For this review, use the dimensioned drawing (mm, ordinates from the lowest corner) and the shaded views. A direction names the side the tool comes from. Coordinates: 2 decimals unless noted, no trailing zeros. Order: outer loops, then holes, each group sorted by start corner. A loop starts at its lowest first (then second) coordinate and runs counter-clockwise, first axis right, second up. Notation, with made-up numbers: M 18.25,15.25 L 53.25,15.25 A21 ccw 53.25,36.25 Z; hole C 62.25,12 d2. An arc over 180 degrees is marked long. One line per item, written item: value.
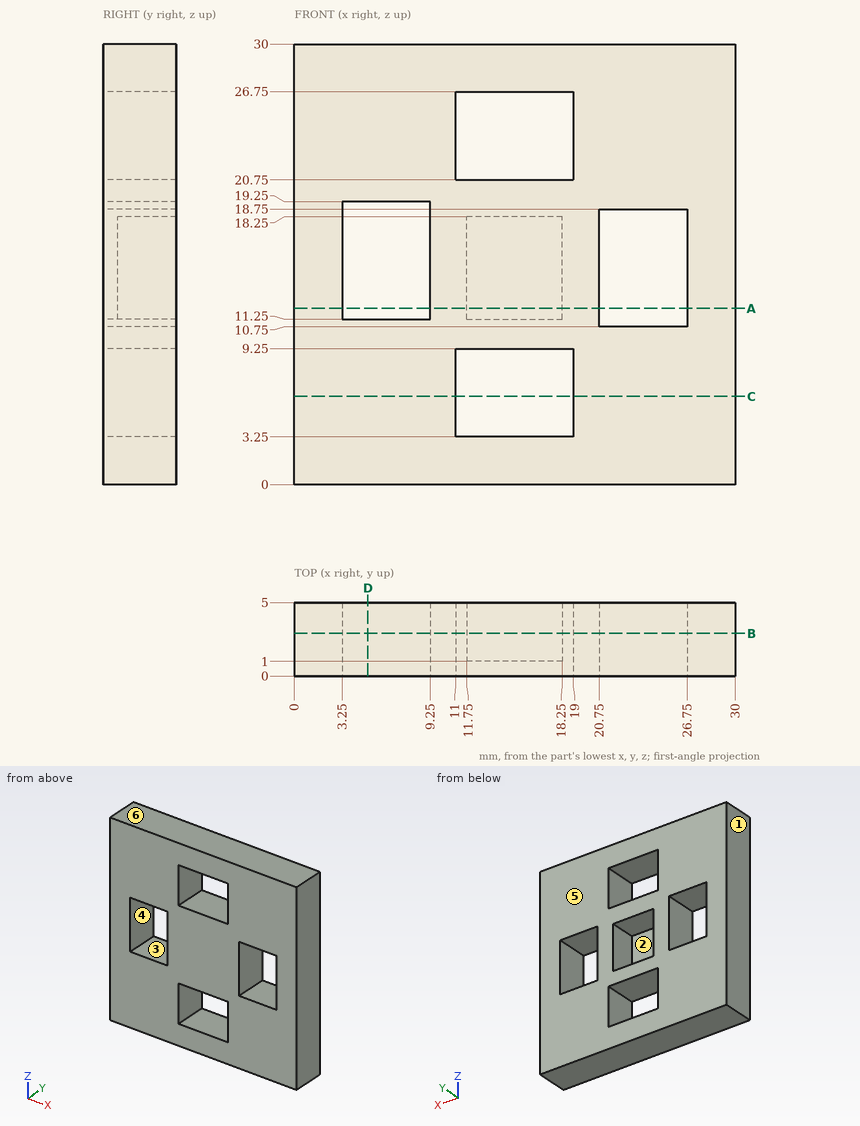
(1) We need section B-B, the plane y = 2.9. State the section outline as (x, z) points.
Geometry results:
outline: M 0,0 L 30,0 L 30,30 L 0,30 Z; hole M 3.25,11.25 L 9.25,11.25 L 9.25,19.25 L 3.25,19.25 Z; hole M 11,3.25 L 19,3.25 L 19,9.25 L 11,9.25 Z; hole M 11,20.75 L 19,20.75 L 19,26.75 L 11,26.75 Z; hole M 11.75,11.25 L 18.25,11.25 L 18.25,18.25 L 11.75,18.25 Z; hole M 20.75,10.75 L 26.75,10.75 L 26.75,18.75 L 20.75,18.75 Z
(2) We need section A-A, the plane z = 12. State the section outline as (x, y) points, plus the area to 3 significant figures.
Geometry results:
outline: M 0,0 L 3.25,0 L 3.25,5 L 0,5 Z; M 9.25,0 L 20.75,0 L 20.75,5 L 18.25,5 L 18.25,1 L 11.75,1 L 11.75,5 L 9.25,5 Z; M 26.75,0 L 30,0 L 30,5 L 26.75,5 Z
area: 64.0 mm2
(3) Tool access review of the marked faces 1, 2 and 3: name each direction out of +Z, -Z, +X, -X, +Y, -Y from which nothing blocks a thin tool from reaching the whole face with its end or side.
Geometry results:
face 1: +Z, -Z, -X, +Y, -Y
face 2: +Y
face 3: +Y, -Y
(4) We need section C-C, the plane z = 6. State the section outline as (x, y) points, plus the area to 3 significant figures.
Geometry results:
outline: M 0,0 L 11,0 L 11,5 L 0,5 Z; M 19,0 L 30,0 L 30,5 L 19,5 Z
area: 110 mm2
(5) Mouldability with a two-part tool opening along Z and no side actions: class the marked faces 4, 5 and 6 as +Z half, -Z half, draft (parallel to the pull), parting line (faces both ways), or undercut.
Geometry results:
face 4: undercut
face 5: draft
face 6: +Z half
(6) For L1, parallel to Z at x = 17, y = 3.25; L2, parallel to X at y = 2.25, z = 16; L3, parallel to Z at x = 13.75, y = 0.75, list the stretches that pass through material, from the lowest coordinate up.
Geometry results:
L1: z = 0 to 3.25, 9.25 to 11.25, 18.25 to 20.75, 26.75 to 30
L2: x = 0 to 3.25, 9.25 to 11.75, 18.25 to 20.75, 26.75 to 30
L3: z = 0 to 3.25, 9.25 to 20.75, 26.75 to 30
(7) We need section D-D, the plane x = 5. State the section outline as (y, z) points, plus the area to 3 significant figures.
Geometry results:
outline: M 0,0 L 5,0 L 5,11.25 L 0,11.25 Z; M 0,19.25 L 5,19.25 L 5,30 L 0,30 Z
area: 110 mm2
